from build123d import *

# Parameters (mm, degrees)
BOSS_EXTRUDE1_DEPTH      = 12.7
BOSS_EXTRUDE1_DEPTH_BACK = 12.7
SKETCH1_R                = 4.064
SKETCH9_W                = 30.48
SKETCH9_H                = 35.052
CUT_EXTRUDE6_DEPTH       = 60.613097773
BOSS_EXTRUDE3_DEPTH      = 12.7
SKETCH11_W               = 5.350768363
SKETCH11_H               = 57.15
CUT_EXTRUDE7_DEPTH       = 75.08914513
SKETCH12_W               = 12.7
SKETCH12_H               = 19.05
CUT_EXTRUDE8_DEPTH       = 89.211973463
SKETCH14_R               = 1.6
CUT_EXTRUDE9_DEPTH       = 75.795998583
SKETCH15_R               = 3.429
CUT_EXTRUDE10_DEPTH      = 75.795998583
CUT_EXTRUDE11_DEPTH      = 2.778125
F_6_CLEARANCE_HOLE1_D    = 3.7973
SKETCH23_R               = 3.175
CUT_EXTRUDE12_DEPTH      = 22.225
CUT_EXTRUDE13_REACH      = 68.032
SKETCH24_W               = 12.7
SKETCH24_H               = 19.05


with BuildPart() as part:
    # Sketch1 → Boss-Extrude1 (new, two sides: drawn at the far end of the back side and taken through both)
    with BuildSketch(Plane.XY.offset(-BOSS_EXTRUDE1_DEPTH_BACK)):
        with BuildLine():
            Line((-26.940768363, -17.415768363), (-26.940768363, 39.734231637))
            Line((-26.940768363, 39.734231637), (26.940768363, 39.734231637))
            Line((26.940768363, 39.734231637), (26.940768363, -17.415768363))
            ThreePointArc((26.940768363, -17.415768363), (36.465768363, -26.940768363), (26.940768363, -36.465768363))
            Line((26.940768363, -36.465768363), (-26.940768363, -36.465768363))
            ThreePointArc((-26.940768363, -36.465768363), (-36.465768363, -26.940768363), (-26.940768363, -17.415768363))
        make_face()
        with Locations((-26.940768363, -26.940768363)):
            Circle(SKETCH1_R, mode=Mode.SUBTRACT)
        with Locations((26.940768363, -26.940768363)):
            Circle(SKETCH1_R, mode=Mode.SUBTRACT)
    extrude(amount=BOSS_EXTRUDE1_DEPTH + BOSS_EXTRUDE1_DEPTH_BACK)

    # Sketch9 → Cut-Extrude6 (cut, through all)
    with BuildSketch(Plane.XY.offset(12.7)):
        with Locations((0, 22.208231637)):
            Rectangle(SKETCH9_W, SKETCH9_H)
    extrude(amount=-CUT_EXTRUDE6_DEPTH, mode=Mode.SUBTRACT)

    # Sketch10 → Boss-Extrude3 (add)
    with BuildSketch(Plane.XY.offset(12.7)):
        Polygon((-26.940768363, 39.734231637), (-26.940768363, -1.667768363), (26.940768363, -1.667768363), (26.940768363, 39.734231637), (15.24, 39.734231637), (15.24, 4.682231637), (-15.24, 4.682231637), (-15.24, 39.734231637), align=None)
    boss_extrude3 = extrude(amount=BOSS_EXTRUDE3_DEPTH)

    # Mirror4: Boss-Extrude3 across plane
    add(boss_extrude3.mirror(Plane.XY))

    # Sketch11 → Cut-Extrude7 (cut, through all)
    with BuildSketch(Plane.XY.offset(25.4)):
        with Locations((-24.265384181, 11.159231637)):
            Rectangle(SKETCH11_W, SKETCH11_H)
    cut_extrude7 = extrude(amount=-CUT_EXTRUDE7_DEPTH, mode=Mode.SUBTRACT)

    # Mirror5: Cut-Extrude7 across plane
    add(cut_extrude7.mirror(Plane(origin=(0, 0, 0), x_dir=(0, 0, 1), z_dir=(1, 0, 0))), mode=Mode.SUBTRACT)

    # Sketch12 → Cut-Extrude8 (cut, through all)
    with BuildSketch(Plane.XZ.offset(36.465768363)):
        Rectangle(SKETCH12_W, SKETCH12_H)
    extrude(amount=-CUT_EXTRUDE8_DEPTH, mode=Mode.SUBTRACT)

    # Sketch14 → Cut-Extrude9 (cut, through all)
    with BuildSketch(Plane.ZY.offset(21.59)):
        with Locations(Location((-18.4, 22.462231637, 0), (0, 0, 90))):
            Circle(SKETCH14_R)
    cut_extrude9 = extrude(amount=-CUT_EXTRUDE9_DEPTH, mode=Mode.SUBTRACT)

    # Mirror6: Cut-Extrude9 across plane
    add(cut_extrude9.mirror(Plane.XY), mode=Mode.SUBTRACT)

    # Sketch15 → Cut-Extrude10 (cut, through all)
    with BuildSketch(Plane(origin=(21.59, 0, 0), x_dir=(0, 0, -1), z_dir=(1, 0, 0))):
        with Locations(Location((0, 22.462231637, 0), (0, 0, 90))):
            Circle(SKETCH15_R)
    extrude(amount=-CUT_EXTRUDE10_DEPTH, mode=Mode.SUBTRACT)

    # Sketch18 → Cut-Extrude11 (cut)
    with BuildSketch(Plane(origin=(0, 4.682231637, 0), x_dir=(1, 0, 0), z_dir=(0, 1, 0))):
        Polygon((-6.35, 2.346351494), (-10.414, 4.692702988), (-14.478, 2.346351494), (-14.478, -2.346351494), (-10.414, -4.692702988), (-6.35, -2.346351494), align=None)
    cut_extrude11 = extrude(amount=-CUT_EXTRUDE11_DEPTH, mode=Mode.SUBTRACT)

    # Mirror7: Cut-Extrude11 across plane
    add(cut_extrude11.mirror(Plane(origin=(0, 0, 0), x_dir=(0, 0, 1), z_dir=(1, 0, 0))), mode=Mode.SUBTRACT)

    # 6 Clearance Hole1 (through all)
    with Locations(Plane(origin=(0, 1.904106637, 0), x_dir=(1, 0, 0), z_dir=(0, 1, 0))):
        with Locations((-10.414, 0)):
            f_6_clearance_hole1 = Hole(F_6_CLEARANCE_HOLE1_D / 2)

    # Mirror8: 6 Clearance Hole1 across plane
    add(f_6_clearance_hole1.mirror(Plane(origin=(0, 0, 0), x_dir=(0, 0, 1), z_dir=(1, 0, 0))), mode=Mode.SUBTRACT)

    # Sketch23 → Cut-Extrude12 (cut)
    with BuildSketch(Plane.XZ.offset(36.465768363)):
        with Locations(Location((-10.414, 0, 0), (0, 0, 270))):
            Circle(SKETCH23_R)
        with Locations(Location((10.414, 0, 0), (0, 0, 270))):
            Circle(SKETCH23_R)
    extrude(amount=-CUT_EXTRUDE12_DEPTH, mode=Mode.SUBTRACT)

    # Sketch24 → Cut-Extrude13 (cut, up to next)
    with BuildSketch(Plane(origin=(0, 0, -12.7), x_dir=(-1, 0, 0), z_dir=(0, 0, -1)), mode=Mode.PRIVATE) as cut_extrude13_sk1:
        with Locations((0, -20.717768363)):
            Rectangle(SKETCH24_W, SKETCH24_H)
    cut_extrude13_tool1 = extrude(cut_extrude13_sk1.sketch, amount=-CUT_EXTRUDE13_REACH, mode=Mode.PRIVATE) & part.part
    add(cut_extrude13_tool1.solids().sort_by_distance((0, -20.717768, -12.7))[0], mode=Mode.SUBTRACT)


solid = part.part
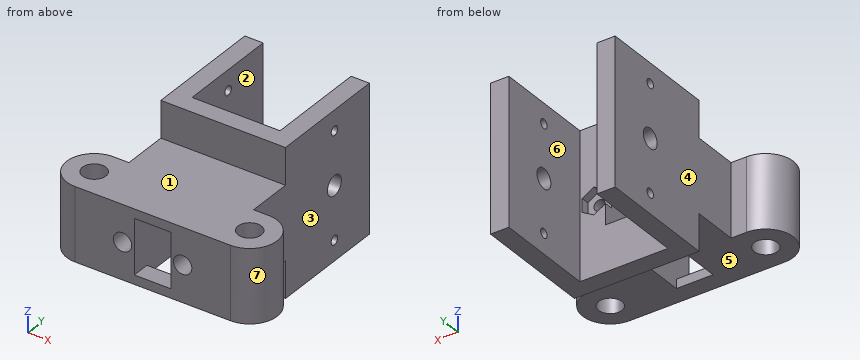
CAD build for the part. Positions are in the model's coordinates, mm. Face numbers are marked on the shaded views. A direction names the side the tool comes from. Coordinates: 2 decimals unless noted, no trailing zeros. Write each loop counter-clockwise with the first axis right and the second up, starting at its lowest first coordinate (ties: lowest second). Pieces come first, ordered by that corner, then holes. Notation, with made-up numbers: M 33.25,46 L 59.25,46 A33 cw 59.25,80 Z; hole C 54.25,86.25 d7. An arc over 180 degrees is marked long. Answer as a JSON object with one key per item and string values. Group by question number.
1) Saw through at D-D (z = 18.4). Write the cut outline in (x, y).
2) Mould opens along X. For the marked faces 5, 6 and 7 say: +X half, -X half, draft (parallel to the pull), parting line (faces both ways), or undercut.
3) Saw through at B-B (x = 3). Write the cut outline in (y, z) (3 decimals).
4) Saw through at C-C (y = 12). Write the cut outline in (x, z).
5) Tool access for the marked faces 1, 2, 3 and 4: list every direction of +Z, -Z, +X, -X, +Y, -Y with a clear straight run to the whole face (end or side of a thin tool).
6) Saw through at A-A (z = -8). Write the cut outline in (x, y) (3 decimals).
7) Wall check: line 1 (X direction, y = 25.5, z = 22); line 2 (Y direction, x = 18, z = -18.4); line 3 (X direction, y = -1, z = 23). Give the ranges that are in metal, low to high. Write a range as from..to.
8) Pin check, flat tips, straight feed: pin 1 Ø0.8 at (y, z) = (3, 0) entering from +X; pin 2 Ø1.5 at (x, z) = (-10.5, 1) entering from -Y; pin 3 Ø8 at (x, z) = (26, 6.5) entering from +Y; pin 4 Ø1 at (x, z) = (-1, -11) entering from +Y. Stop position of each tip, or through.
Values follow:
{
 "1": {"outline": "M -21.59,-1.67 L 21.59,-1.67 L 21.59,20.86 L 15.24,20.86 L 15.24,4.68 L -15.24,4.68 L -15.24,20.86 L -21.59,20.86 Z; M -21.59,24.06 L -15.24,24.06 L -15.24,39.73 L -21.59,39.73 Z; M 15.24,24.06 L 21.59,24.06 L 21.59,39.73 L 15.24,39.73 Z"},
 "2": {"face 5": "draft", "face 6": "undercut", "face 7": "+X half"},
 "3": {"outline": "M -36.466,-12.7 L -30.243,-12.7 L -30.243,-9.525 L -36.466,-9.525 Z; M -36.466,9.525 L 4.682,9.525 L 4.682,25.4 L -1.668,25.4 L -1.668,12.7 L -36.466,12.7 Z; M -11.193,-12.7 L -1.668,-12.7 L -1.668,-25.4 L 4.682,-25.4 L 4.682,-9.525 L -11.193,-9.525 Z"},
 "4": {"outline": "M -21.59,-25.4 L -15.24,-25.4 L -15.24,25.4 L -21.59,25.4 Z; M 15.24,-25.4 L 21.59,-25.4 L 21.59,25.4 L 15.24,25.4 Z"},
 "5": {"face 1": "+Z, +X, -X, -Y", "face 2": "+Z, -Z, +Y", "face 3": "+Z, -Z, +X, +Y", "face 4": "+Z, -Z, -X, +Y"},
 "6": {"outline": "M -26.941,-36.466 L -6.35,-36.466 L -6.35,4.682 L -15.24,4.682 L -15.24,39.734 L -21.59,39.734 L -21.59,-17.416 L -26.941,-17.416 A9.525 ccw Z; M 6.35,-36.466 L 26.941,-36.466 A9.525 ccw 26.941,-17.416 L 21.59,-17.416 L 21.59,39.734 L 15.24,39.734 L 15.24,4.682 L 6.35,4.682 Z; hole C -26.941,-26.941 d8.128; hole C 26.941,-26.941 d8.128"},
 "7": {"line 1": "x = -21.59..-15.24, 15.24..21.59", "line 2": "y = -1.67..20.86, 24.06..39.73", "line 3": "x = -21.59..21.59"},
 "8": {"pin 1": "stops at x = 21.59", "pin 2": "passes through", "pin 3": "stops at y = -17.42", "pin 4": "stops at y = 4.68"}
}
